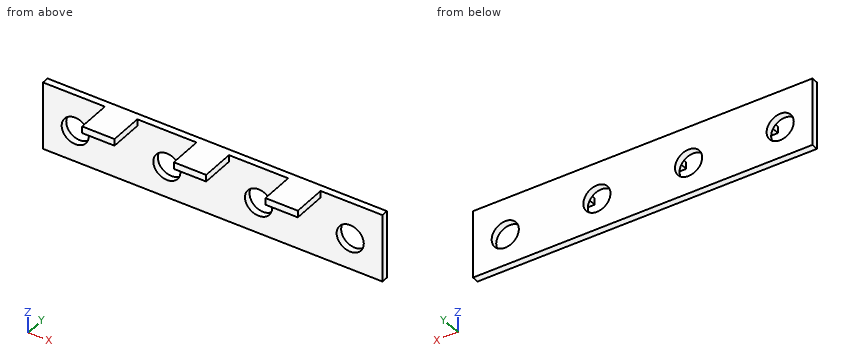
from build123d import *

# Parameters (mm, degrees)
SKETCH1_W           = 127
SKETCH1_H           = 25.4
SKETCH1_R           = 5.08
BOSS_EXTRUDE1_DEPTH = 2.54
SKETCH2_W           = 127
SKETCH2_H           = 2.54
BOSS_EXTRUDE2_DEPTH = 12.7
SKETCH4_W           = 23.145
SKETCH4_H           = 12.7
SKETCH4_W_2         = 22.16
CUT_EXTRUDE1_DEPTH  = 2.54


with BuildPart() as part:
    # Sketch1 → Boss-Extrude1 (new body)
    with BuildSketch(Plane(origin=(0, 0, 0), x_dir=(1, 0, 0), z_dir=(0, 1, 0))):
        with Locations((63.5, 12.7)):
            Rectangle(SKETCH1_W, SKETCH1_H)
        with Locations(Location((12.065, 13.716, 0), (0, 0, 270))):
            Circle(SKETCH1_R, mode=Mode.SUBTRACT)
        with Locations(Location((46.355, 13.716, 0), (0, 0, 270))):
            Circle(SKETCH1_R, mode=Mode.SUBTRACT)
        with Locations(Location((80.645, 13.716, 0), (0, 0, 270))):
            Circle(SKETCH1_R, mode=Mode.SUBTRACT)
        with Locations(Location((114.935, 13.716, 0), (0, 0, 270))):
            Circle(SKETCH1_R, mode=Mode.SUBTRACT)
    extrude(amount=BOSS_EXTRUDE1_DEPTH)

    # Sketch2 → Boss-Extrude2 (add)
    with BuildSketch(Plane.XZ):
        with Locations((63.5, -1.27)):
            Rectangle(SKETCH2_W, SKETCH2_H)
    extrude(amount=BOSS_EXTRUDE2_DEPTH)

    # Sketch4 → Cut-Extrude1 (cut)
    with BuildSketch(Plane(origin=(0, 0, -2.54), x_dir=(-1, 0, 0), z_dir=(0, 0, -1))):
        with Locations((-115.4275, -6.35)):
            Rectangle(SKETCH4_W, SKETCH4_H)
        with Locations((-80.645, -6.35)):
            Rectangle(SKETCH4_W_2, SKETCH4_H)
        with Locations((-46.355, -6.35)):
            Rectangle(SKETCH4_W_2, SKETCH4_H)
        with Locations((-11.5725, -6.35)):
            Rectangle(SKETCH4_W, SKETCH4_H)
    extrude(amount=-CUT_EXTRUDE1_DEPTH, mode=Mode.SUBTRACT)


solid = part.part
Could you check a few things on this model? Use its own coordinates, in mm. Coordinates: 2 decimals unless noted, no trailing zeros. Order: outer loops, then holes, each group sorted by start corner. A loop starts at its lowest first (then second) coordinate and runs counter-clockwise, first axis right, second up.
Q1. Suppose I cut it at D-D on x = 34. Please give me the cut outline in (y, z), and give its area (3 significant figures).
Q2. Will these pins go through, and if not, where does the flat tip stop? pin 1 (8 mm diameter, centred on y = -6.5, z = -14.5, fed in from +X); pin 2 (3 mm diameter, centred on y = -3.5, z = -1.5, fed in from +X) (3 decimals); pin 3 (0.8 mm diameter, centred on y = -5, z = -1.5, fed in from -X) (3 decimals); pin 4 (13 mm diameter, centred on x = 12.065, z = -13.716, fed in from -Y).
Q3. Please list where these lines run through material, in increasing order: L1, parallel to X at y = -6.25, z = -2.5 (3 decimals); L2, parallel to Y at x = 29, z = -23.5; L3, parallel to X at y = 2, z = -16.
Q4. Suppose I cut it at A-A on y = -6.75. Please give me the cut outline in (x, z) (3 decimals).
Q5. Suppose I cut it at B-B on x = 79. Please give me the cut outline in (y, z), and give its area (3 significant figures).
Q6. Suppose I cut it at C-C on z = -15.5. Please give me the cut outline in (x, y), and give its area (3 significant figures).
Answer:
1. outline: (-12.7, -2.54) - (0, -2.54) - (0, -25.4) - (2.54, -25.4) - (2.54, 0) - (-12.7, 0) - close
1. area: 96.8 mm2
2. pin 1: passes through
2. pin 2: stops at x = 103.855
2. pin 3: stops at x = 23.145
2. pin 4: stops at y = 0
3. L1: x = 23.145 to 35.275, 57.435 to 69.565, 91.725 to 103.855
3. L2: y = 0 to 2.54
3. L3: x = 0 to 7.53, 16.6 to 41.82, 50.89 to 76.11, 85.18 to 110.4, 119.47 to 127
4. outline: (23.145, -2.54) - (35.275, -2.54) - (35.275, 0) - (23.145, 0) - close; (57.435, -2.54) - (69.565, -2.54) - (69.565, 0) - (57.435, 0) - close; (91.725, -2.54) - (103.855, -2.54) - (103.855, 0) - (91.725, 0) - close
5. outline: (0, -25.4) - (2.54, -25.4) - (2.54, -18.52) - (0, -18.52) - close; (0, -8.91) - (2.54, -8.91) - (2.54, 0) - (0, 0) - close
5. area: 40.1 mm2
6. outline: (0, 0) - (7.31, 0) - (7.31, 2.54) - (0, 2.54) - close; (16.82, 0) - (41.6, 0) - (41.6, 2.54) - (16.82, 2.54) - close; (51.11, 0) - (75.89, 0) - (75.89, 2.54) - (51.11, 2.54) - close; (85.4, 0) - (110.18, 0) - (110.18, 2.54) - (85.4, 2.54) - close; (119.69, 0) - (127, 0) - (127, 2.54) - (119.69, 2.54) - close
6. area: 226 mm2
